from build123d import *

# Parameters (mm, degrees)
SKETCH4_R           = 1
CUT_EXTRUDE3_DEPTH  = 43.380808577
SKETCH6_R           = 65
SKETCH6_R_2         = 55
BOSS_EXTRUDE1_DEPTH = 10


with BuildPart() as part:
    # Sketch2 → Revolve1 (revolve)
    with BuildSketch(Plane.XY):
        with BuildLine():
            Line((0, -88.845849199), (0, -72))
            ThreePointArc((0, -72), (-30.319276667, -65.304988036), (-55, -46.465040622))
            Line((-55, -46.465040622), (-65, -46.465040622))
            Line((-65, -46.465040622), (-65, -88.845849199))
            Line((-65, -88.845849199), (-55, -88.845849199))
            Line((-55, -88.845849199), (0, -88.845849199))
        make_face()
    revolve(axis=Axis((0, -72, 0), (0, -1, 0)))

    # Sketch4 → Cut-Extrude3 (cut, through all)
    with BuildSketch(Plane.XZ.offset(88.845849199)):
        Circle(SKETCH4_R)
        with Locations((25, 0)):
            Circle(SKETCH4_R)
        with Locations((12.5, -21.650635095)):
            Circle(SKETCH4_R)
        with Locations((-12.5, -21.650635095)):
            Circle(SKETCH4_R)
        with Locations((-25, 0)):
            Circle(SKETCH4_R)
        with Locations((-12.5, 21.650635095)):
            Circle(SKETCH4_R)
        with Locations((12.5, 21.650635095)):
            Circle(SKETCH4_R)
    extrude(amount=-CUT_EXTRUDE3_DEPTH, mode=Mode.SUBTRACT)

    # Sketch6 → Boss-Extrude1 (add)
    with BuildSketch(Plane.XZ.offset(88.845849199)):
        Circle(SKETCH6_R)
        Circle(SKETCH6_R_2, mode=Mode.SUBTRACT)
    extrude(amount=BOSS_EXTRUDE1_DEPTH)


solid = part.part
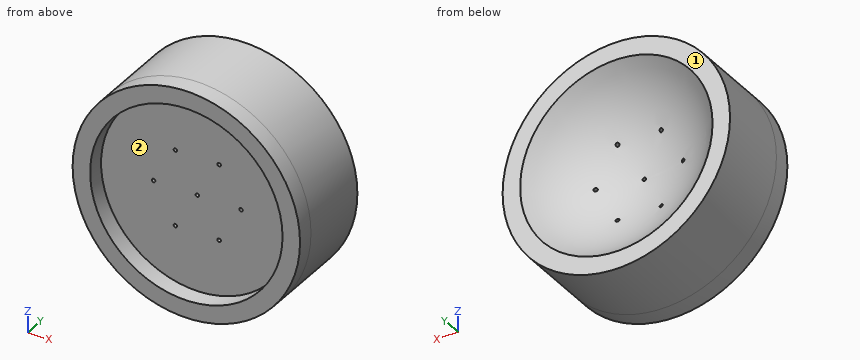
Input: part model. Units: mm. Frame: model coordinates. Face numbers are marked on the shaded views. Coordinates: 2 decimals unless noted, no trailing zeros. Loops run counter-clockwise (first coordinate to the right, second up) from the corner with the lowest first, then second, coordinate; pieces in that order, holes last.
(1) Section B-B on x = 52. Return the cut outline in (y, z), then the cut area to 3 significant figures.
(2) Section C-C on z = -33.5. Return the cut outline in (x, y).
(3) First-contact query: pin 1 Ø10 at (x, z) = (41, -17.5) entering from -Y; pin 2 Ø2 at (x, y) = (0, -67.5) entering from -Z; pin 3 Ø5 at (x, y) = (14.5, -75.5) entering from +Z. Flat tips, straight axial feed; report the tip coordinate or a pass-through.
(4) Pull-direction query (X, two-part tool) for the marked faces 1 and 2; classes: released by +X, released by -X, zero draft, split by the parting line, or undercut.
(5) Section A-A on y = -75.5. Return the cut outline in (x, z).
(6) Material intervals for probe 1 along Z at (x, y) = (12.5, -77); probe 2 along Z at (x, y) = (0, -77.5); probe 3 along Z at (x, y) = (12, -81), sorted ascending.
(7) Section D-D on y = -91. Return the cut outline in (x, z).
Data:
1. outline: (-98.85, -39) - (-46.47, -39) - (-46.47, -17.92) arc R49.8 cw to (-46.47, 17.92) - (-46.47, 39) - (-98.85, 39) - (-98.85, 17.92) - (-88.85, 17.92) - (-88.85, -17.92) - (-98.85, -17.92) - close
1. area: 3,650 mm2
2. outline: (-55.7, -98.85) - (-43.62, -98.85) - (-43.62, -88.85) - (43.62, -88.85) - (43.62, -98.85) - (55.7, -98.85) - (55.7, -46.47) - (43.62, -46.47) arc R63.73 cw to (-43.62, -46.47) - (-55.7, -46.47) - close
3. pin 1: stops at y = -88.85
3. pin 2: stops at z = -65
3. pin 3: stops at z = 63.88
4. face 1: zero draft
4. face 2: undercut
5. outline: circle Ø130 at (0, 0); hole circle Ø2 at (-25, 0); hole circle Ø2 at (-12.5, -21.65); hole circle Ø2 at (-12.5, 21.65); hole circle Ø2 at (0, 0); hole circle Ø2 at (12.5, -21.65); hole circle Ø2 at (12.5, 21.65); hole circle Ø2 at (25, 0)
6. probe 1: z = -63.79 to -22.65, -20.65 to 20.65, 22.65 to 63.79
6. probe 2: z = -65 to -1, 1 to 65
6. probe 3: z = -63.88 to -22.52, -20.78 to 20.78, 22.52 to 63.88
7. outline: circle Ø130 at (0, 0); hole circle Ø110 at (0, 0)
